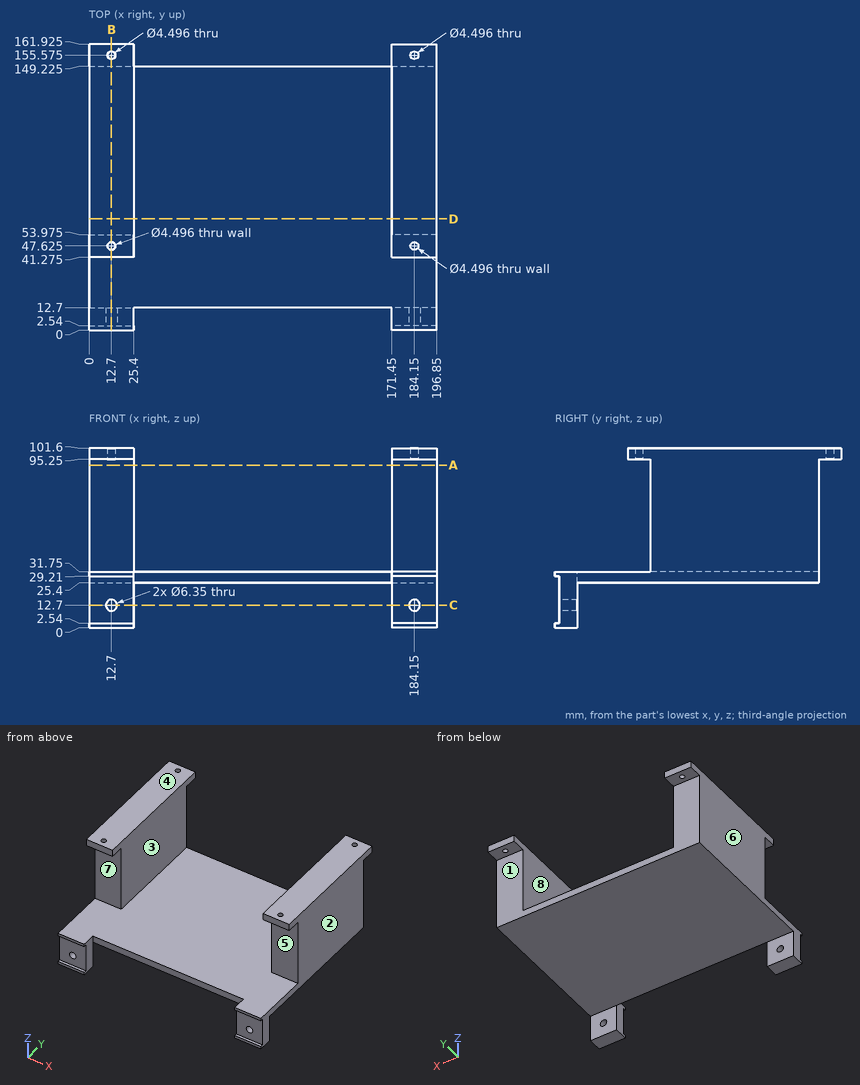
Geometry: see drawing. Coordinates: mm, zero at the bounding-box minimum. A direction names the side the tool comes from. Coordinates: 2 decimals unless noted, no trailing zeros. Loops run counter-clockwise (first coordinate to the right, second up) from the corner with the lowest first, then second, coordinate; pieces in that order, holes last.
Q1. Cut plane D-D (y = 63). Output: boundary loops of the cut face in (x, z).
Q2. Material intervals for line 1 (Y direction, x = 184.15, z = 100.75) (1 decimal); line 2 (X direction, y = 59, z = 87); line 3 (Z direction, x = 184, y = 6), sorted ascending.
Q3. Cut plane A-A (z = 92). Output: boundary loops of the cut face in (x, y) (3 decimals), then the cut area to 3 significant figures.
Q4. Cut plane B-B (x = 12.7). Give the number of separate pieces and of enclosed holes in the cut face, then the cut area to 3 significant figures.
Q5. Contact query for flat-ended pins moving along their axis: pin 1 (10 mm diameter, centred on x = 180, y = 49.5, fed in from -Z); pin 2 (4 mm diameter, centred on x = 190, y = 157.5, fed in from -Z); pin 3 (3 mm diameter, centred on x = 104, y = 27.5, fed in from +Z); pin 4 (5 mm diameter, centred on x = 12.7, z = 12.7, fed in from +Y). Output: stop coordinate, or through.
Q6. Cut plane C-C (z = 12.7). Output: boundary loops of the cut face in (x, y) (3 decimals).
Q7. Set-up query: the marked faces 1, 2, 3, 4 and 5. Return all of +Z, -Z, +X, -X, +Y, -Y with unobstructed straight access to the full face (end or side cutting, diameter ignored); none if empty.
Q8. Draft query along X for the marked faces 6, 7 and 8. Return one class per face: +X half, -X half, draft (parallel to the pull), parting line (faces both ways), or undercut.
Working result:
1. outline: (0, 25.4) - (196.85, 25.4) - (196.85, 101.6) - (171.45, 101.6) - (171.45, 31.75) - (25.4, 31.75) - (25.4, 101.6) - (0, 101.6) - close
2. line 1: y = 41.3 to 45.4, 49.9 to 153.3, 157.8 to 161.9
2. line 2: x = 0 to 25.4, 171.45 to 196.85
2. line 3: z = 0 to 9.53, 15.87 to 31.75
3. outline: (0, 53.975) - (25.4, 53.975) - (25.4, 149.225) - (0, 149.225) - close; (171.45, 53.975) - (196.85, 53.975) - (196.85, 149.225) - (171.45, 149.225) - close
3. area: 4,840 mm2
4. separate pieces: 4
4. enclosed holes: 0
4. area: 7,900 mm2
5. pin 1: stops at z = 25.4
5. pin 2: stops at z = 95.25
5. pin 3: stops at z = 31.75
5. pin 4: passes through
6. outline: (0, 2.54) - (9.525, 2.54) - (9.525, 12.7) - (0, 12.7) - close; (15.875, 2.54) - (25.4, 2.54) - (25.4, 12.7) - (15.875, 12.7) - close; (171.45, 2.54) - (180.975, 2.54) - (180.975, 12.7) - (171.45, 12.7) - close; (187.325, 2.54) - (196.85, 2.54) - (196.85, 12.7) - (187.325, 12.7) - close
7. face 1: -Z, +X, -X, +Y
7. face 2: +Z, -Z, +X, +Y, -Y
7. face 3: +Z, +Y, -Y
7. face 4: +Z, +X, -X, +Y, -Y
7. face 5: +X, -X, -Y
8. face 6: -X half
8. face 7: draft
8. face 8: undercut
